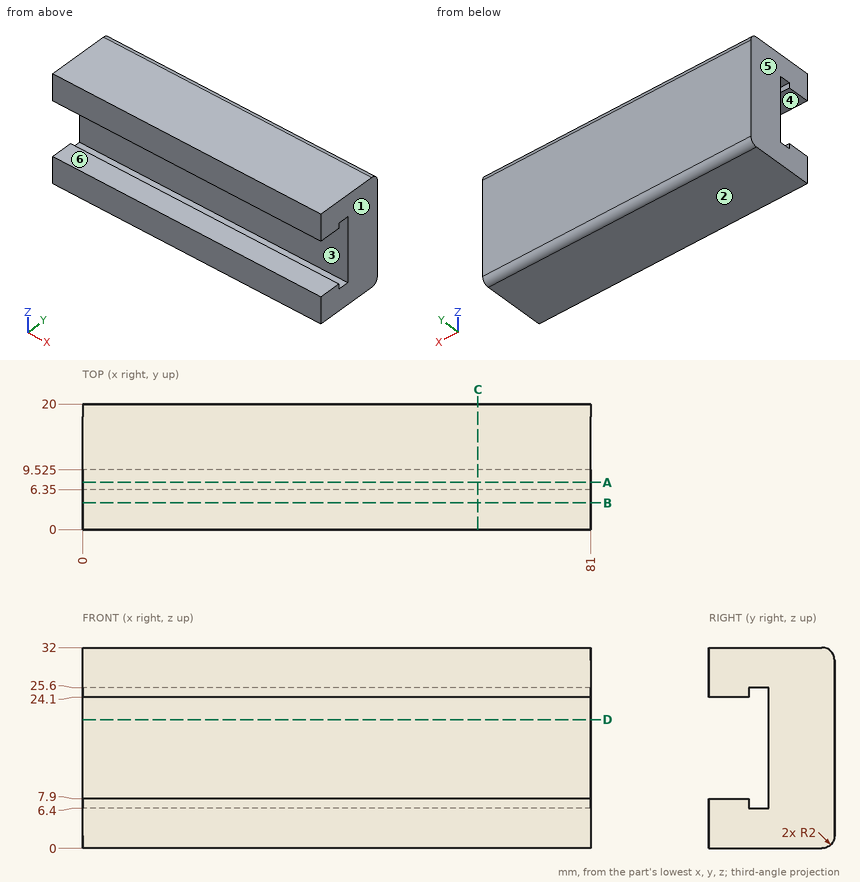
Drawing for the job (mm, zero at the part's lowest x, y, z). A direction names the side the tool comes from. Round coordinates to 2 decimals unless told otherwise and drop trailing zeros. Loops run counter-clockwise (first coordinate to the right, second up) from the corner with the lowest first, then second, coordinate; pieces in that order, holes last. Notation, with made-up numbers: (85, 34) -> (111, 34) arc R16 cw to (111, 63) -> close; hole circle Ø3 at (21, 61). An arc over 180 degrees is marked (long way). Use one line per item in the form item = value. Start each with the question number.
Item 1: Band-saw the part on C-C (x = 63). List the corners of the cut face in (y, z) (3 decimals).
Item 2: Band-saw the part on B-B (y = 4.25). List the corners of the cut face in (x, z).
Item 3: Drop a flat-ended pin along its axis: pin 1 Ø5 at (x, z) = (37.5, 20) entering from -Y (3 decimals). Give the stop position or say it passes through.
Item 4: Band-saw the part on A-A (y = 7.5). List the corners of the cut face in (x, z), plus the area to 3 significant figures.
Item 5: Band-saw the part on D-D (z = 20.5). List the corners of the cut face in (x, y) (3 decimals).
Item 6: Drill centre lines: line 1 along Z through (x, y) = (57.5, 6.5); line 2 along Y through (x, z) = (51, 25) (3 decimals); line 3 along Z through (x, y) = (57, 5). Where is each one in solid material? Low to high.
Item 7: Tool access for the marked faces 5 and 6: list every direction of +Z, -Z, +X, -X, +Y, -Y with a clear straight run to the whole face (end or side of a thin tool).
Item 8: Two-plate mould, pull along Z, no slides. Class the marked faces 1, 2, 3 and 4: released by +Z, released by -Z, zero draft, split by the parting line, or undercut.
Data:
q1.outline = (0, 0) -> (18, 0) arc R2 ccw to (20, 2) -> (20, 30) arc R2 ccw to (18, 32) -> (0, 32) -> (0, 24.1) -> (6.35, 24.1) -> (6.35, 25.6) -> (9.525, 25.6) -> (9.525, 6.4) -> (6.35, 6.4) -> (6.35, 7.9) -> (0, 7.9) -> close
q2.outline = (0, 0) -> (81, 0) -> (81, 7.9) -> (0, 7.9) -> close; (0, 24.1) -> (81, 24.1) -> (81, 32) -> (0, 32) -> close
q3.pin_1 = 9.525
q4.outline = (0, 0) -> (81, 0) -> (81, 6.4) -> (0, 6.4) -> close; (0, 25.6) -> (81, 25.6) -> (81, 32) -> (0, 32) -> close
q4.area = 1,040 mm^2
q5.outline = (0, 9.525) -> (81, 9.525) -> (81, 20) -> (0, 20) -> close
q6.line_1 = 0 to 6.4, 25.6 to 32
q6.line_2 = 0 to 6.35, 9.525 to 20
q6.line_3 = 0 to 7.9, 24.1 to 32
q7.face_5 = +Z, -Z, -X, +Y, -Y
q7.face_6 = +X, -X, -Y
q8.face_1 = zero draft
q8.face_2 = released by -Z
q8.face_3 = undercut
q8.face_4 = undercut
